```python
from build123d import *

# Parameters (mm, degrees)
SKETCH1_W           = 100
SKETCH1_H           = 100
BOSS_EXTRUDE1_DEPTH = 10
SKETCH2_R           = 2
CUT_EXTRUDE1_DEPTH  = 72.414284285
CUT_EXTRUDE2_DEPTH  = 4
SKETCH4_R           = 5
CUT_EXTRUDE3_DEPTH  = 71.964779997
SKETCH5_R           = 7.65
SKETCH5_R_2         = 5.15
EXTRUDE_THIN1_DEPTH = 20
RIB6_START          = -1.5
RIB6_DEPTH          = 3
CIRPATTERN2_COUNT   = 4
FILLET1_R           = 5


with BuildPart() as part:
    # Sketch1 → Boss-Extrude1 (new body)
    with BuildSketch(Plane(origin=(0, 0, 0), x_dir=(1, 0, 0), z_dir=(0, 1, 0))):
        Rectangle(SKETCH1_W, SKETCH1_H)
    extrude(amount=BOSS_EXTRUDE1_DEPTH)

    # Sketch2 → Cut-Extrude1 (cut, through all)
    with BuildSketch(Plane(origin=(0, 10, 0), x_dir=(1, 0, 0), z_dir=(0, 1, 0))):
        with Locations(Location((-45, 35, 0), (0, 0, 270))):
            Circle(SKETCH2_R)
        with Locations(Location((45, 35, 0), (0, 0, 270))):
            Circle(SKETCH2_R)
        with Locations(Location((45, -35, 0), (0, 0, 270))):
            Circle(SKETCH2_R)
        with Locations(Location((-45, -35, 0), (0, 0, 270))):
            Circle(SKETCH2_R)
    extrude(amount=-CUT_EXTRUDE1_DEPTH, mode=Mode.SUBTRACT)

    # Sketch3 → Cut-Extrude2 (cut)
    with BuildSketch(Plane.XZ):
        Polygon((-20.762395693, 0), (-25.381197846, 8), (-34.618802154, 8), (-39.237604307, 0), (-34.618802154, -8), (-25.381197846, -8), align=None)
        Polygon((25.381197846, -8), (20.762395693, 0), (25.381197846, 8), (34.618802154, 8), (39.237604307, 0), (34.618802154, -8), align=None)
    extrude(amount=-CUT_EXTRUDE2_DEPTH, mode=Mode.SUBTRACT)

    # Sketch4 → Cut-Extrude3 (cut, through all)
    with BuildSketch(Plane.XZ.offset(-4)):
        with Locations(Location((-30, 0, 0), (0, 0, 270))):
            Circle(SKETCH4_R)
        with Locations(Location((30, 0, 0), (0, 0, 90))):
            Circle(SKETCH4_R)
    extrude(amount=-CUT_EXTRUDE3_DEPTH, mode=Mode.SUBTRACT)

    # Sketch5 → Extrude-Thin1 (add)
    with BuildSketch(Plane.XZ):
        Circle(SKETCH5_R)
        Circle(SKETCH5_R_2, mode=Mode.SUBTRACT)
    extrude(amount=EXTRUDE_THIN1_DEPTH)

    # Rib6: read off the stored shape, not the designer's step
    # Rib6 outline → Rib6 (add)
    with BuildSketch(Plane(origin=(0, 0, 0), x_dir=(0.7071067811865461, 0, -0.7071067811865489), z_dir=(0.7071067811865489, 0, 0.7071067811865461)).offset(RIB6_START)):
        Polygon((7.65, -20), (22.65, 0), (7.50149985, 0), (7.50149985, -20), align=None)
    rib6 = extrude(amount=RIB6_DEPTH)

    # CirPattern2: Rib6 ×4 about axis
    cirpattern2_axis = Axis((0, 0, 0), (0, 1, 0))
    for i in range(1, CIRPATTERN2_COUNT):
        add(rib6.rotate(cirpattern2_axis, i * 360 / CIRPATTERN2_COUNT))

    # Fillet1
    fillet1_edges = [part.edges().sort_by_distance(p)[0] for p in [
        (50, 5, 50),
        (-50, 5, 50),
        (-50, 5, -50),
        (50, 5, -50),
    ]]
    fillet(fillet1_edges, radius=FILLET1_R)


solid = part.part
```
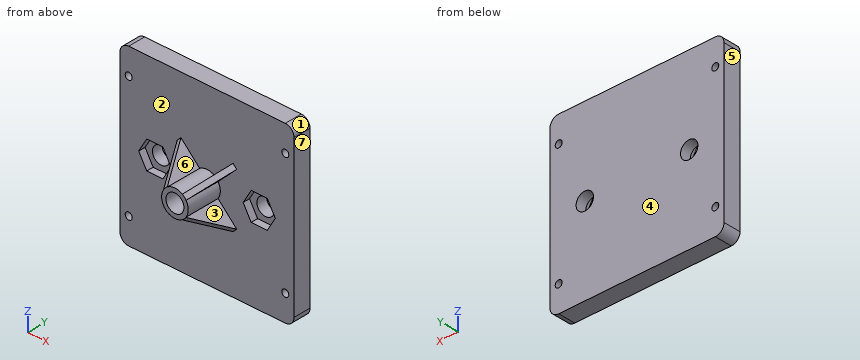
Check sheet for the modelled part. Datum: model origin and axes. Units: mm. Face numbers are marked on the shaded views. A direction names the side the tool comes from. Give positions to 0.01 mm unless a question says otherwise; leave off trailing zeros. Order: outer loops, then holes, each group sorted by start corner. A loop starts at its lowest first (then second) coordinate and runs counter-clockwise, first axis right, second up. Notation, with made-up numbers: M 20,1.5 L 70,1.5 A3 cw 70,5.5 Z; hole C -36.75,28.5 d4. An arc over 180 degrees is marked long. Answer in a Markdown table with one row per item. Add a question column.
Q1. Sectioned sample at C-C, the plane x = 30. Record the boundary of the cut face in (y, z).
Q2. Thickness scan on L1, parallel to X at y = 4.5, z = -35; L2, parallel to X at y = 6.25, z = 0; L3, parallel to Y at x = 41, z = -35. Record the ranges inside material, lowest first.
Q3. Gauge pin test, flat ends, axial feed: pin 1 Ø12 at (x, z) = (34, 24) entering from -Y; pin 2 Ø1.5 at (y, z) = (-12, -7) entering from -X; pin 3 Ø8 at (y, z) = (-5, -9) entering from +X; pin 4 Ø6 at (x, z) = (-30, 0) entering from +Y. Record the tip position at first contact, or that the pin passes through.
Q4. Sectioned sample at B-B, the plane z = -35. Record the boundary of the cut face in (x, y).
Q5. Sectioned sample at D-D, the plane y = -2. Record the boundary of the cut face in (x, z), and give its area (3 significant figures).
Q6. Sectioned sample at A-A, the plane y = 6.75. Record the boundary of the cut face in (x, z).
Q7. Access from +Z, -Z, +X, -X, +Y, -Y to the whole of each face (thin tool, end or side, straight path). Record for the marked faces 1, 2 and 3.
Q8. Release check for a two-part mould opening along X. For the marked faces 4, 5, 6 and 7 record: released by +X, released by -X, zero draft, split by the parting line, or undercut.
Verdict:
| question | item | result |
|---|---|---|
| 1 | outline | M 0,-50 L 10,-50 L 10,-5 L 4,-5 L 4,-8 L 0,-8 Z; M 0,8 L 4,8 L 4,5 L 10,5 L 10,50 L 0,50 Z |
| 2 | L1 | -50 to -47, -43 to 43, 47 to 50 |
| 2 | L2 | -50 to -35, -25 to 25, 35 to 50 |
| 2 | L3 | 0 to 10 |
| 3 | pin 1 | y = 0 |
| 3 | pin 2 | x = -9.87 |
| 3 | pin 3 | x = 14.98 |
| 3 | pin 4 | through |
| 4 | outline | M -50,0 L -47,0 L -47,10 L -50,10 Z; M -43,0 L 43,0 L 43,10 L -43,10 Z; M 47,0 L 50,0 L 50,10 L 47,10 Z |
| 5 | outline | M -16.02,-13.89 L -13.89,-16.02 L -4.24,-6.37 A7.65 ccw 4.24,-6.37 L 13.89,-16.02 L 16.02,-13.89 L 6.37,-4.24 A7.65 ccw 6.37,4.24 L 16.02,13.89 L 13.89,16.02 L 4.24,6.37 A7.65 ccw -4.24,6.37 L -13.89,16.02 L -16.02,13.89 L -6.37,4.24 A7.65 ccw -6.37,-4.24 Z; hole C 0,0 d10.3 |
| 5 | area | 263 mm² |
| 6 | outline | M -50,-45 A5 ccw -45,-50 L 45,-50 A5 ccw 50,-45 L 50,45 A5 ccw 45,50 L -45,50 A5 ccw -50,45 Z; hole C -45,-35 d4; hole C -45,35 d4; hole C -30,0 d10; hole C 30,0 d10; hole C 45,-35 d4; hole C 45,35 d4 |
| 7 | face 1 | +Z, +X, +Y, -Y |
| 7 | face 2 | -Y |
| 7 | face 3 | +X, -Y |
| 8 | face 4 | zero draft |
| 8 | face 5 | released by -X |
| 8 | face 6 | undercut |
| 8 | face 7 | released by +X |
